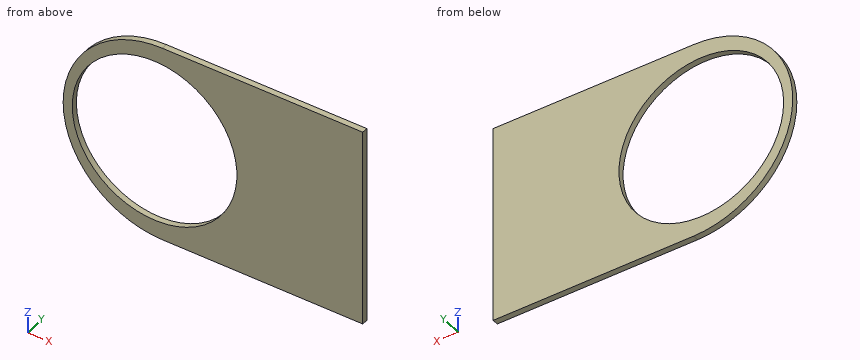
```python
from build123d import *

# Parameters (mm, degrees)
F2_DEPTH = 3
F3_D     = 83


with BuildPart() as f2:
    # F0 (on Front) → F2 (new body)
    with BuildSketch(Plane.XZ):
        with BuildLine():
            Line((-21.7263168246, 58.1104420125), (-122.7263168246, 57.9687414691))
            ThreePointArc((-122.7263168246, 57.9687414691), (-172.7263168246, 7.9687414691), (-122.7263168246, -42.0312585309))
            Line((-122.7263168246, -42.0312585309), (-21.7263168246, -42.0312585309))
            Line((-21.7263168246, -42.0312585309), (-21.7263168246, 57.9687414691))
            Line((-21.7263168246, 57.9687414691), (-21.7263168246, 57.9720512033))
            Line((-21.7263168246, 57.9720512033), (-21.7263168246, 58.1104420125))
        make_face()
    extrude(amount=F2_DEPTH)

    # F3 (through all)
    with Locations(Plane(origin=(0, 0, 0), x_dir=(1, 0, 0), z_dir=(0, 1, 0))):
        with Locations((-126.6402751207, -7.990530692)):
            Hole(F3_D / 2)


solid = f2.part
```
Could you check a few things on this model? Use its own coordinates, in mm. Coordinates: 2 decimals unless noted, no trailing zeros. Write each loop counter-clockwise with the first axis right and the second up, starting at its lowest first coordinate (ties: lowest second). Pieces come first, ordered by that corner, then holes. Notation, with made-up numbers: (13, -17) -> (34, -17) arc R22 ccw to (34, 14) -> close; hole circle Ø5 at (71, 50.5). An arc over 180 degrees is marked (long way). One line per question, with ' | ' between items. Start each with the question number.
1. If we section it at C-C (y = -1.1): Please give me the cut outline in (x, z).
2. If we section it at B-B (z = 25.5): Please give me the cut outline in (x, y).
3. Please list where these lines run through material, in increasing order: line 1 along Z through (x, y) = (-99.5, -1.95); line 2 along Z through (x, y) = (-98.5, -1.25); line 3 along X through (y, z) = (-0.6, 18.5).
4. If we section it at A-A (x = -99.5): Please give me the cut outline in (y, z), and give its area (3 significant figures).
Return value:
1) outline: (-122.73, -42.03) -> (-21.73, -42.03) -> (-21.73, 58.11) -> (-122.73, 57.97) arc R50 ccw to start; hole circle Ø83 at (-126.64, 7.99)
2) outline: (-169.55, -3) -> (-164.27, -3) -> (-164.27, 0) -> (-169.55, 0) -> close; (-89.01, -3) -> (-21.73, -3) -> (-21.73, 0) -> (-89.01, 0) -> close
3) line 1: z = -42.03 to -23.4, 39.39 to 58 | line 2: z = -42.03 to -22.51, 38.49 to 58 | line 3: x = -171.6 to -166.79, -86.49 to -21.73
4) outline: (-3, -42.03) -> (0, -42.03) -> (0, -23.4) -> (-3, -23.4) -> close; (-3, 39.39) -> (0, 39.39) -> (0, 58) -> (-3, 58) -> close | area: 112 mm²
